For this review, take the finished solid that the model builds, in its own axes (mm). A direction names the side the tool comes from. Give positions to 0.01 mm unless a question says otherwise; leave off trailing zeros. Write each loop counter-clockwise with the first axis right and the second up, starting at its lowest first coordinate (ties: lowest second). Pieces come first, ordered by that corner, then holes.
1) We need section A-A on z = 11.5. Give the boundary of the cut face in (x, y), and give its area (3 significant figures).
2) We need section B-B on x = 7. Give the boundary of the cut face in (y, z), and give its area (3 significant figures).
3) Machinability: for faces 4 (the face through (15, 10, 6)), 5 (the face through (12.4, 17.43, 6.16)), which of the approach directions +Z, -Z, +X, -X, +Y, -Y give a long, thin tool a straight path to every point of the face, cutting with its end or side? Answer none if there is none.
4) We need section C-C on y = 15. Give the boundary of the cut face in (x, z).
5) We need section D-D on y = 18.75. Give the boundary of the cut face in (x, z).
6) Wall thickness on line 1 along X through (y, z) = (5.25, 10.75); line 2 along Y through (x, z) = (7.5, 7.5); line 3 along Y through (x, z) = (12.25, 3.5): over which ranges is each line inside the solid? List them lowest first.
7) Draft analysis for pull direction Y (two halves, no side actions). For faces 1 (the face through (14.4, 0.57, 6.16)), 2 (the face through (2.6, 2.57, 6.16)), 3 (the face through (0.6, 19.43, 6.16)), state which applies: pulls with the +Y half, pulls with the -Y half, needs draft (parallel to the pull), parting line crosses it, or undercut.
from build123d import *

# Parameters (mm, degrees)
F1_DEPTH = 12.5


with BuildPart() as f1:
    # F0 (on Top) → F1 (new body)
    with BuildSketch(Plane.XY):
        with BuildLine():
            ThreePointArc((0, 2), (0.585786, 0.585786), (2, 0))
            Line((2, 0), (13, 0))
            ThreePointArc((13, 0), (14.414214, 0.585786), (15, 2))
            Line((15, 2), (15, 18))
            ThreePointArc((15, 18), (14.414214, 19.414214), (13, 20))
            Line((13, 20), (2, 20))
            ThreePointArc((2, 20), (0.585786, 19.414214), (0, 18))
            Line((0, 18), (0, 2))
        make_face()
        with BuildLine():
            ThreePointArc((2, 16), (2.585786, 17.414214), (4, 18))
            Line((4, 18), (11, 18))
            ThreePointArc((11, 18), (12.414214, 17.414214), (13, 16))
            Line((13, 16), (13, 4))
            ThreePointArc((13, 4), (12.414214, 2.585786), (11, 2))
            Line((11, 2), (4, 2))
            ThreePointArc((4, 2), (2.585786, 2.585786), (2, 4))
            Line((2, 4), (2, 16))
        make_face(mode=Mode.SUBTRACT)
    extrude(amount=F1_DEPTH)


solid = f1.part
Results list:
1. outline: (0, 2) arc R2 ccw to (2, 0) - (13, 0) arc R2 ccw to (15, 2) - (15, 18) arc R2 ccw to (13, 20) - (2, 20) arc R2 ccw to (0, 18) - close; hole (2, 4) arc R2 ccw to (4, 2) - (11, 2) arc R2 ccw to (13, 4) - (13, 16) arc R2 ccw to (11, 18) - (4, 18) arc R2 ccw to (2, 16) - close
1. area: 124 mm2
2. outline: (0, 0) - (2, 0) - (2, 12.5) - (0, 12.5) - close; (18, 0) - (20, 0) - (20, 12.5) - (18, 12.5) - close
2. area: 50.0 mm2
3. face 4: +Z, -Z, +X, +Y, -Y
3. face 5: +Z, -Z
4. outline: (0, 0) - (2, 0) - (2, 12.5) - (0, 12.5) - close; (13, 0) - (15, 0) - (15, 12.5) - (13, 12.5) - close
5. outline: (0.15, 0) - (14.85, 0) - (14.85, 12.5) - (0.15, 12.5) - close
6. line 1: x = 0 to 2, 13 to 15
6. line 2: y = 0 to 2, 18 to 20
6. line 3: y = 0 to 2.44, 17.56 to 20
7. face 1: pulls with the -Y half
7. face 2: undercut
7. face 3: pulls with the +Y half
